Read the model definition and answer for the solid it produces. Units are mm, in the model's axes. Face numbers are marked on the shaded views. Coordinates: 2 decimals unless noted, no trailing zeros. Loops run counter-clockwise (first coordinate to the right, second up) from the corner with the lowest first, then second, coordinate; pieces in that order, holes last.
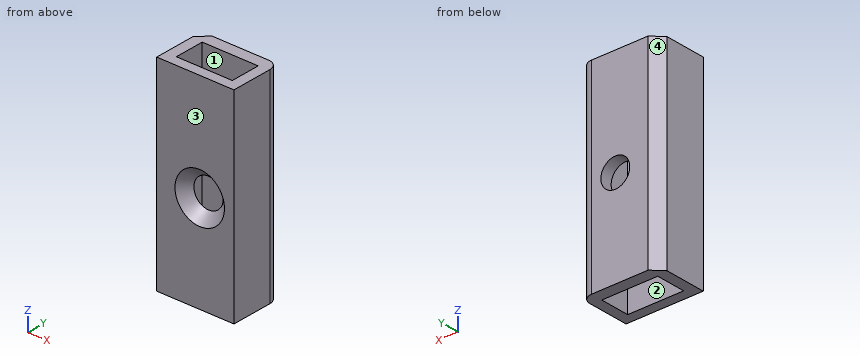
from build123d import *

# Parameters (mm, degrees)
F0_W     = 38.0692742765
F0_H     = 25.5331452936
F1_DEPTH = 100
F2_DEPTH = 23.622
F3_R     = 7.1236409115
F4_DEPTH = 56.642
F5_R     = 5.08
F6_SIZE  = 5.08
F7_SIZE  = 5
F8_W     = 27.580646798
F8_H     = 14.6975801326
F9_DEPTH = 109.9


with BuildPart() as f1:
    # F0 (on Top) → F1 (new body)
    with BuildSketch(Plane.XY):
        with Locations((19.0346371382, 12.7665726468)):
            Rectangle(F0_W, F0_H)
    extrude(amount=F1_DEPTH)

    # F2 (add): a face of the model
    f2_faces = [f1.faces().sort_by_distance(p)[0] for p in [
        (38.0692742765, 12.7665726468, 50),
    ]]
    extrude(f2_faces, amount=-F2_DEPTH)

    # F3 (on face) → F4 (cut)
    with BuildSketch(Plane(origin=(0, 25.5331452936, 0), x_dir=(-1, 0, 0), z_dir=(0, 1, 0))):
        with Locations((-21.2079435587, 47.6018153131)):
            Circle(F3_R)
    extrude(amount=-F4_DEPTH, mode=Mode.SUBTRACT)

    # F5
    f5_edges = [f1.edges().sort_by_distance(p)[0] for p in [
        (38.069274, 25.533145, 50),
    ]]
    fillet(f5_edges, radius=F5_R)

    # F6
    f6_edges = [f1.edges().sort_by_distance(p)[0] for p in [
        (28.331584, 0, 47.601815),
    ]]
    chamfer(f6_edges, length=F6_SIZE)

    # F7
    f7_edges = [f1.edges().sort_by_distance(p)[0] for p in [
        (0, 25.533145, 50),
    ]]
    chamfer(f7_edges, length=F7_SIZE)

    # F8 (on face) → F9 (cut)
    with BuildSketch(Plane.XY.offset(100)):
        with Locations((19.1431464627, 12.3387097847)):
            Rectangle(F8_W, F8_H)
    extrude(amount=-F9_DEPTH, mode=Mode.SUBTRACT)


solid = f1.part
Item 1: A cutting plane is placed at D-D on y = 1.5. Determine the outline of the cut face in (x, z), then the cut area to 3 significant figures.
Numbers:
outline: (0, 0) - (38.07, 0) - (38.07, 100) - (0, 100) - close; hole circle Ø21.41 at (21.21, 47.6)
area: 3,450 mm2
Item 2: Find the intervals of material crossed by line 1 along Y through (x, z) = (6, 59); line 2 along X through (y, z) = (6, 32); line 3 along Y through (x, z) = (17.5, 39), in increasing order.
Numbers:
line 1: y = 0 to 4.99, 19.69 to 25.53
line 2: x = 0 to 5.35, 32.93 to 38.07
line 3: y = 2.84 to 4.99, 19.69 to 25.53
Item 3: Given pin 1 (8.5 mm diameter, centred on x = 17, z = 52, fed in from +Y); pin 2 (8.5 mm diameter, centred on x = 21.21, z = 47.6, fed in from -Y); pin 3 (8.5 mm diameter, centred on x = 20.5, z = 43, fed in from -Y), each flat-ended and moving along its own axis, determine where each tip first touches the part or whether it passes through.
Numbers:
pin 1: stops at y = 25.53
pin 2: passes through
pin 3: stops at y = 3.3
Item 4: A cutting plane is placed at C-C on z = 29. Determine the outline of the cut face in (x, y), then the cut area to 3 significant figures.
Numbers:
outline: (0, 0) - (38.07, 0) - (38.07, 20.45) arc R5.08 ccw to (32.99, 25.53) - (5, 25.53) - (0, 20.53) - close; hole (5.35, 4.99) - (32.93, 4.99) - (32.93, 19.69) - (5.35, 19.69) - close
area: 549 mm2
Item 5: A cutting plane is placed at B-B on x = 6.5. Determine the outline of the cut face in (y, z), then the cut area to 3 significant figures.
Numbers:
outline: (0, 0) - (4.99, 0) - (4.99, 100) - (0, 100) - close; (19.69, 0) - (25.53, 0) - (25.53, 100) - (19.69, 100) - close
area: 1,080 mm2
Item 6: A cutting plane is placed at A-A on y = 11.25. Determine the outline of the cut face in (x, z), then the cut area to 3 significant figures.
Numbers:
outline: (0, 0) - (5.35, 0) - (5.35, 100) - (0, 100) - close; (32.93, 0) - (38.07, 0) - (38.07, 100) - (32.93, 100) - close
area: 1,050 mm2
Item 7: Determine the mould class of the marked faces 1, 2, 3 and 4 for opening direction Y: released by +Y, released by -Y, zero draft, split by the parting line, or undercut.
Numbers:
face 1: undercut
face 2: undercut
face 3: released by -Y
face 4: released by +Y
